from build123d import *

# Parameters (mm, degrees)
ESQUISSE1_W             = 275
ESQUISSE1_H             = 145
ESQUISSE1_R             = 10.5
ESQUISSE1_R_2           = 8
BOSS_EXTRU_1_DEPTH      = 10
ESQUISSE2_W             = 275
ESQUISSE2_H             = 95
BOSS_EXTRU_2_DEPTH      = 125
ESQUISSE4_R             = 10.5
ENL_V_MAT_EXTRU_1_DEPTH = 317.662280671


with BuildPart() as part:
    # Esquisse1 → Boss.-Extru.1 (new body)
    with BuildSketch(Plane.XY):
        with Locations((137.5, 72.5)):
            Rectangle(ESQUISSE1_W, ESQUISSE1_H)
        with Locations((60, 123)):
            Circle(ESQUISSE1_R, mode=Mode.SUBTRACT)
        with Locations((25, 85)):
            Circle(ESQUISSE1_R_2, mode=Mode.SUBTRACT)
        with Locations(Location((250, 85, 0), (0, 0, 180))):
            Circle(ESQUISSE1_R_2, mode=Mode.SUBTRACT)
        with Locations(Location((215, 123, 0), (0, 0, 180))):
            Circle(ESQUISSE1_R, mode=Mode.SUBTRACT)
    extrude(amount=BOSS_EXTRU_1_DEPTH)

    # Esquisse2 → Boss.-Extru.2 (add)
    with BuildSketch(Plane(origin=(0, 0, 0), x_dir=(1, 0, 0), z_dir=(0, 1, 0))):
        with Locations((137.5, -47.5)):
            Rectangle(ESQUISSE2_W, ESQUISSE2_H)
    extrude(amount=BOSS_EXTRU_2_DEPTH)

    # Esquisse4 → Enlèv. mat.-Extru.1 (cut, through all)
    with BuildSketch(Plane(origin=(0, 125, 0), x_dir=(1, 0, 0), z_dir=(0, 1, 0))):
        with Locations(Location((206.25, -52.5, 0), (0, 0, 270))):
            Circle(ESQUISSE4_R)
        with Locations(Location((137.5, -52.5, 0), (0, 0, 270))):
            Circle(ESQUISSE4_R)
        with Locations(Location((68.75, -52.5, 0), (0, 0, 270))):
            Circle(ESQUISSE4_R)
    extrude(amount=-ENL_V_MAT_EXTRU_1_DEPTH, mode=Mode.SUBTRACT)


solid = part.part
Source: CAD feature listing. Evaluate the final solid. Frame: model axes, mm. A direction names the side the tool comes from. Coordinates: 2 decimals unless noted, no trailing zeros. Loops run counter-clockwise (first coordinate to the right, second up) from the corner with the lowest first, then second, coordinate; pieces in that order, holes last. Notation, with made-up numbers: (-39, 49) -> (20, 49) arc R15 cw to (20, 58) -> close; hole circle Ø4 at (46, 33.5). An arc over 180 degrees is marked (long way). Answer in a Markdown table with one row per item. Add a question column.
Q1. Section B-B on y = 19.5. Return the cut outline in (x, z).
Q2. Section C-C on x = 137.5. Return the cut outline in (y, z).
Q3. Ray query, line 1 along X through (y, z) = (28.5, 52.5); line 2 along X through (y, z) = (9, 55); line 3 along Z through (x, y) = (137, 39). Return the intervals inside material, ascending.
Q4. Pull-direction query (X, two-part tool) for faces 1 (the face through (0, 71, 48)), 2 (the face through (75.846, 63.375, 44.761)), 3 (the face through (131.11, 63.38, 44.17)), 4 (the face through (136, 0, 36)); classes: pulls with the +X half, pulls with the -X half, needs draft (parallel to the pull), parting line crosses it, or undercut.
Q5. Reachability of faces 5 (the face through (136, 135, 10)), 6 (the face through (213.346, 63.375, 44.761)) from +Z, -Z, +X, -X, +Y, -Y: full face, straight path, thin tool, end or side. Return the list, or none.
Q6. Section A-A on z = 52.5. Return the cut outline in (x, y).
Q7. Section D-D on x = 221.5. Return the cut outline in (y, z).
Q8. Contact query for flat-ended pins moving along their axis: pin 1 Ø24 at (x, z) = (206.25, 52.5) entering from -Y; pin 2 Ø1 at (x, z) = (45, 39) entering from +Y; pin 3 Ø6 at (x, y) = (177, 133.5) entering from +Z. Output: stop coordinate, or through.
Computed values:
| question | item | result |
|---|---|---|
| 1 | outline | (0, 0) -> (275, 0) -> (275, 95) -> (0, 95) -> close; hole circle Ø21 at (68.75, 52.5); hole circle Ø21 at (137.5, 52.5); hole circle Ø21 at (206.25, 52.5) |
| 2 | outline | (0, 0) -> (145, 0) -> (145, 10) -> (125, 10) -> (125, 42) -> (0, 42) -> close; (0, 63) -> (125, 63) -> (125, 95) -> (0, 95) -> close |
| 3 | line 1 | x = 0 to 58.25, 79.25 to 127, 148 to 195.75, 216.75 to 275 |
| 3 | line 2 | x = 0 to 58.55, 78.95 to 127.3, 147.7 to 196.05, 216.45 to 275 |
| 3 | line 3 | z = 0 to 42.01, 62.99 to 95 |
| 4 | face 1 | pulls with the -X half |
| 4 | face 2 | undercut |
| 4 | face 3 | undercut |
| 4 | face 4 | needs draft |
| 5 | face 5 | +Z, +X, -X, +Y |
| 5 | face 6 | +Y, -Y |
| 6 | outline | (0, 0) -> (58.25, 0) -> (58.25, 125) -> (0, 125) -> close; (79.25, 0) -> (127, 0) -> (127, 125) -> (79.25, 125) -> close; (148, 0) -> (195.75, 0) -> (195.75, 125) -> (148, 125) -> close; (216.75, 0) -> (275, 0) -> (275, 125) -> (216.75, 125) -> close |
| 7 | outline | (0, 0) -> (125, 0) -> (125, 95) -> (0, 95) -> close; (131.25, 0) -> (145, 0) -> (145, 10) -> (131.25, 10) -> close |
| 8 | pin 1 | stops at y = 0 |
| 8 | pin 2 | stops at y = 125 |
| 8 | pin 3 | stops at z = 10 |
